Here's how the part is built. I have some questions about the finished solid (model axes, mm). Face numbers are marked on the shaded views. A direction names the side the tool comes from. Coordinates: 2 decimals unless noted, no trailing zeros. Order: outer loops, then holes, each group sorted by start corner. A loop starts at its lowest first (then second) coordinate and runs counter-clockwise, first axis right, second up. Notation, with made-up numbers: (-35, -28) - (9, -28) arc R11 ccw to (9, -17) - close; hole circle Ø3 at (17, -30.75). An arc over 180 degrees is marked (long way). Answer in a Markdown table with one row per item. Add a question column.
Item 1: I want a section at A-A (z = 11.25). Please give me the cut outline in (x, y), plus the area to 3 significant figures.
Item 2: I want a section at D-D (z = 16.75). Please give me the cut outline in (x, y).
Item 3: I want a section at B-B (x = -4). Please give me the cut outline in (y, z), plus the area to 3 significant figures.
Item 4: Will these pins go through, and if not, where does the flat tip stop? pin 1 Ø9 at (x, z) = (-10, 10) entering from +Y; pin 2 Ø2 at (x, z) = (-5, 4.5) entering from +Y; pin 3 Ø3 at (x, z) = (-17.5, 16) entering from +Y.
Item 5: I want a section at C-C (x = -11). Please give me the cut outline in (y, z), plus the area to 3 significant figures.
Item 6: On a 3-axis mill with a long thin cutter (end or side, diameter ignored), from which of +Z, -Z, +X, -X, +Y, -Y can I reach the whole of each face in a straight line? I mean the marked faces 1, 2 and 3. Say none if no direction works.
Item 7: Thinking about a two-plate mould opening in X: for the marked faces 4, 5 and 6, which applies, +X half, -X half, draft (parallel to the pull), parting line (faces both ways), or undercut?
Item 8: If I drill on line 1 along Z through (x, y) = (-10, -14.25); line 2 along Z through (x, y) = (-1.1, -10); line 3 along Y through (x, z) = (-5.5, 14.5), over which ranges is the centre line in solid material (lowest first)? Write a range as from..to.
```python
from build123d import *

# Parameters (mm, degrees)
BOSS_EXTRU_1_DEPTH      = 20
ESQUISSE2_R             = 3.55
ENL_V_MAT_EXTRU_1_DEPTH = 21
ESQUISSE3_R             = 3.55
ENL_V_MAT_EXTRU_2_DEPTH = 21
ENL_V_START             = -3.5
ESQUISSE4_R             = 5.5
ENL_V_MAT_EXTRU_3_DEPTH = 17.5
ESQUISSE5_R             = 5.5
ENL_V_MAT_EXTRU_4_DEPTH = 17.5
CONG_1_R                = 0.1


with BuildPart() as part:
    # Esquisse1 → Boss.-Extru.1 (new body)
    with BuildSketch(Plane.XY):
        Polygon((-20, -20), (0, 0), (0, -20), align=None)
    extrude(amount=BOSS_EXTRU_1_DEPTH)

    # Esquisse2 → Enlèv. mat.-Extru.1 (cut, through all)
    with BuildSketch(Plane.XZ.offset(20)):
        with Locations((-10, 10)):
            Circle(ESQUISSE2_R)
    extrude(amount=-ENL_V_MAT_EXTRU_1_DEPTH, mode=Mode.SUBTRACT)

    # Esquisse3 → Enlèv. mat.-Extru.2 (cut, through all)
    with BuildSketch(Plane(origin=(0, 0, 0), x_dir=(0, 0, 1), z_dir=(1, 0, 0))):
        with Locations((10, 10)):
            Circle(ESQUISSE3_R)
    extrude(amount=-ENL_V_MAT_EXTRU_2_DEPTH, mode=Mode.SUBTRACT)

    # Esquisse4 → Enlèv. mat.-Extru.3 (cut, through all)
    with BuildSketch(Plane(origin=(0, 0, 0), x_dir=(0, 0, -1), z_dir=(1, 0, 0)).offset(ENL_V_START)):
        with Locations((-10, -10)):
            Circle(ESQUISSE4_R)
    extrude(amount=-ENL_V_MAT_EXTRU_3_DEPTH, mode=Mode.SUBTRACT)

    # Esquisse5 → Enlèv. mat.-Extru.4 (cut, through all)
    with BuildSketch(Plane.XZ.offset(20).offset(ENL_V_START)):
        with Locations((-10, 10)):
            Circle(ESQUISSE5_R)
    extrude(amount=-ENL_V_MAT_EXTRU_4_DEPTH, mode=Mode.SUBTRACT)

    # Congé1
    cong_1_edges = [part.edges().sort_by_distance(p)[0] for p in [
        (-20, -20, 10),
        (0, 0, 10),
    ]]
    fillet(cong_1_edges, radius=CONG_1_R)


solid = part.part
```
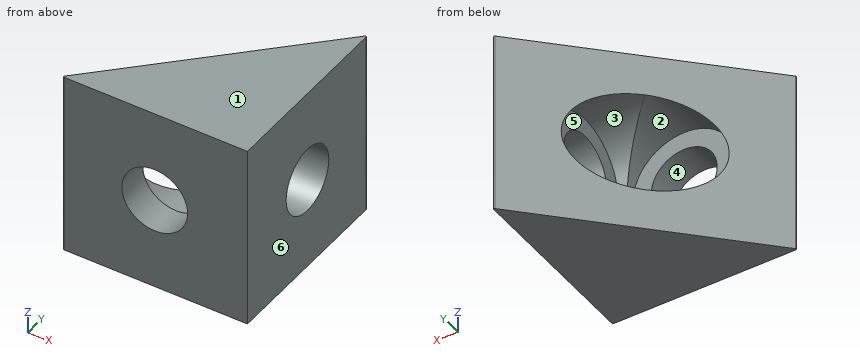
Values follow:
| question | item | result |
|---|---|---|
| 1 | outline | (-19.83, -19.83) arc R0.1 ccw to (-19.76, -20) - (-13.32, -20) - (-13.32, -16.5) - (-15.36, -16.5) - (-15.36, -15.36) - close; (-6.68, -20) - (0, -20) - (0, -13.32) - (-3.5, -13.32) - (-3.5, -15.36) - (-4.64, -15.36) - (-4.64, -16.5) - (-6.68, -16.5) - close; (-4.64, -4.64) - (-3.5, -4.64) - (-3.5, -6.68) - (0, -6.68) - (0, -0.24) arc R0.1 ccw to (-0.17, -0.17) - close |
| 1 | area | 71.6 mm^2 |
| 2 | outline | (-19.83, -19.83) arc R0.1 ccw to (-19.76, -20) - (0, -20) - (0, -0.24) arc R0.1 ccw to (-0.17, -0.17) - close |
| 3 | outline | (-20, 0) - (-4, 0) - (-4, 20) - (-20, 20) - close; hole circle Ø11 at (-10, 10) |
| 3 | area | 225 mm^2 |
| 4 | pin 1 | stops at y = -16.5 |
| 4 | pin 2 | stops at y = -4 |
| 4 | pin 3 | stops at y = -16 |
| 5 | outline | (-20, 0) - (-11, 0) - (-11, 4.59) - (-16.5, 4.59) - (-16.5, 6.59) - (-20, 6.59) - close; (-20, 13.41) - (-16.5, 13.41) - (-16.5, 15.41) - (-11, 15.41) - (-11, 20) - (-20, 20) - close |
| 5 | area | 96.7 mm^2 |
| 6 | face 1 | +Z, +X, -X, +Y, -Y |
| 6 | face 2 | +Y |
| 6 | face 3 | -X |
| 7 | face 4 | undercut |
| 7 | face 5 | -X half |
| 7 | face 6 | +X half |
| 8 | line 1 | z = 0..4.5, 15.5..20 |
| 8 | line 2 | z = 0..6.45, 13.55..20 |
| 8 | line 3 | y = -20..-13.16, -6.84..-5.5 |
